```python
from build123d import *

# Parameters (mm, degrees)
SKETCH1_W   = 145
SKETCH1_H   = 163
SKETCH1_H_2 = 164
BAGA_DEPTH  = 20


with BuildPart() as part:
    # Sketch1 → baga (new body)
    with BuildSketch(Plane(origin=(0, 0, 0), x_dir=(1, 0, 0), z_dir=(0, 1, 0))):
        with BuildLine():
            Line((0, 0), (-680, 0))
            Line((-680, 0), (-680, -520))
            ThreePointArc((-680, -520), (-665.355339059, -555.355339059), (-630, -570))
            Line((-630, -570), (-50, -570))
            ThreePointArc((-50, -570), (-14.644660941, -555.355339059), (0, -520))
            Line((0, -520), (0, 0))
        make_face()
        with Locations((-587.5, -284.5)):
            Rectangle(SKETCH1_W, SKETCH1_H, mode=Mode.SUBTRACT)
        with Locations((-92.5, -101.5)):
            Rectangle(SKETCH1_W, SKETCH1_H, mode=Mode.SUBTRACT)
        with BuildLine():
            Line((-70, -550), (-165, -550))
            Line((-165, -550), (-165, -386))
            Line((-165, -386), (-20, -386))
            Line((-20, -386), (-20, -500))
            ThreePointArc((-20, -500), (-34.644660941, -535.355339059), (-70, -550))
        make_face(mode=Mode.SUBTRACT)
        with Locations((-587.5, -101.5)):
            Rectangle(SKETCH1_W, SKETCH1_H, mode=Mode.SUBTRACT)
        with BuildLine():
            Line((-660, -386), (-515, -386))
            Line((-515, -386), (-515, -550))
            Line((-515, -550), (-610, -550))
            ThreePointArc((-610, -550), (-645.355339059, -535.355339059), (-660, -500))
            Line((-660, -500), (-660, -386))
        make_face(mode=Mode.SUBTRACT)
        with Locations((-422.5, -101.5)):
            Rectangle(SKETCH1_W, SKETCH1_H, mode=Mode.SUBTRACT)
        with Locations((-257.5, -101.5)):
            Rectangle(SKETCH1_W, SKETCH1_H, mode=Mode.SUBTRACT)
        with Locations((-422.5, -284.5)):
            Rectangle(SKETCH1_W, SKETCH1_H, mode=Mode.SUBTRACT)
        with Locations((-257.5, -284.5)):
            Rectangle(SKETCH1_W, SKETCH1_H, mode=Mode.SUBTRACT)
        with Locations((-92.5, -284.5)):
            Rectangle(SKETCH1_W, SKETCH1_H, mode=Mode.SUBTRACT)
        with Locations((-422.5, -468)):
            Rectangle(SKETCH1_W, SKETCH1_H_2, mode=Mode.SUBTRACT)
        with Locations((-257.5, -468)):
            Rectangle(SKETCH1_W, SKETCH1_H_2, mode=Mode.SUBTRACT)
    extrude(amount=BAGA_DEPTH)


solid = part.part
```
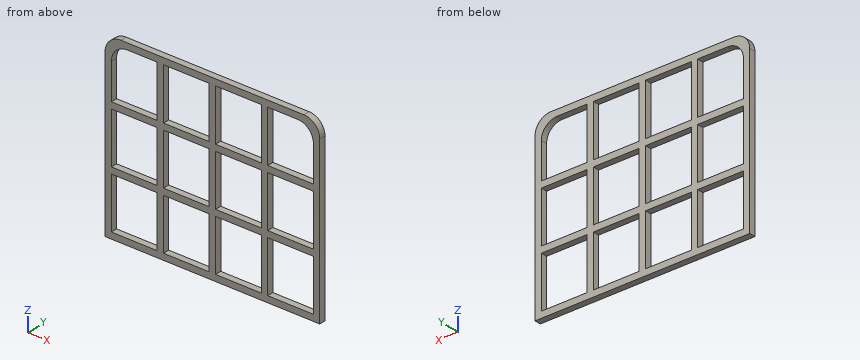
Could you check a few things on this model? Use its own coordinates, in mm. Coordinates: 2 decimals unless noted, no trailing zeros. Write each loop counter-clockwise with the first axis right and the second up, starting at its lowest first coordinate (ties: lowest second). Pieces come first, ordered by that corner, then holes. Notation, with made-up numbers: (-15.5, 1) -> (43.5, 1) arc R22 ccw to (43.5, 8) -> close; hole circle Ø11 at (71, -39). An arc over 180 degrees is marked (long way). Write item = value, one per line. Start each with the question number.
(1) I want a section at D-D (z = 531.5). Please give me the cut outline in (x, y).
(2) I want a section at B-B (z = 220). Please give me the cut outline in (x, y).
(3) I need wall thicknesses on line 1 (X direction, y = 8.5, z = 473); line 2 (Z direction, x = -238, y = 1.5); line 3 (Z direction, x = -645, y = 10.75). Which ranges of each line are inside material? Lowest first, please. Write a range as [from, to].
(4) I want a section at A-A (x = -251.5). Please give me the cut outline in (y, z), plus the area to 3 significant figures.
(5) I want a section at C-C (y = 10.5). Give the number of separate pieces and of enclosed holes in the cut face, plus the area to 3 significant figures.
Result set:
q1.outline = (-678.66, 0) -> (-648.83, 0) -> (-648.83, 20) -> (-678.66, 20) -> close; (-515, 0) -> (-495, 0) -> (-495, 20) -> (-515, 20) -> close; (-350, 0) -> (-330, 0) -> (-330, 20) -> (-350, 20) -> close; (-185, 0) -> (-165, 0) -> (-165, 20) -> (-185, 20) -> close; (-31.17, 0) -> (-1.34, 0) -> (-1.34, 20) -> (-31.17, 20) -> close
q2.outline = (-680, 0) -> (-660, 0) -> (-660, 20) -> (-680, 20) -> close; (-515, 0) -> (-495, 0) -> (-495, 20) -> (-515, 20) -> close; (-350, 0) -> (-330, 0) -> (-330, 20) -> (-350, 20) -> close; (-185, 0) -> (-165, 0) -> (-165, 20) -> (-185, 20) -> close; (-20, 0) -> (0, 0) -> (0, 20) -> (-20, 20) -> close
q3.line_1 = [-680, -660], [-515, -495], [-350, -330], [-185, -165], [-20, 0]
q3.line_2 = [0, 20], [183, 203], [366, 386], [550, 570]
q3.line_3 = [0, 20], [183, 203], [366, 386], [535.71, 567.7]
q4.outline = (0, 0) -> (20, 0) -> (20, 20) -> (0, 20) -> close; (0, 183) -> (20, 183) -> (20, 203) -> (0, 203) -> close; (0, 366) -> (20, 366) -> (20, 386) -> (0, 386) -> close; (0, 550) -> (20, 550) -> (20, 570) -> (0, 570) -> close
q4.area = 1,600 mm2
q5.separate_pieces = 1
q5.enclosed_holes = 12
q5.area = 103,000 mm2
